Solid Edge part; units mm, degrees
sketch "Sketch1" plane through (0, 0, 0) normal (0, 0, 1) x (1, 0, 0)
  circle A0 centre (0, 0) radius 9.135
extrude "Protrusion1" add sketch "Sketch1" along normal blind 9
sketch "Sketch2" plane through (0, 0, 9) normal (0, 0, 1) x (1, 0, 0)
  line L0 (0, -3.4641) -> (-3, -1.7321)
  line L1 (-3, -1.7321) -> (-3, 1.7321)
  line L2 (-3, 1.7321) -> (0, 3.4641)
  line L3 (0, 3.4641) -> (3, 1.7321)
  line L4 (3, 1.7321) -> (3, -1.7321)
  line L5 (3, -1.7321) -> (0, -3.4641)
extrude "Cutout1" cut sketch "Sketch2" against normal blind 4.5
sketch "Sketch3" plane through (0, 0, 0) normal (0, 0, -1) x (0, 1, 0)
  circle A0 centre (0, 0) radius 6
extrude "Protrusion2" add sketch "Sketch3" along normal blind 25
sketch "Sketch4" plane through (0, 0, -25) normal (0, 0, -1) x (0, 1, 0)
  circle A0 centre (0, 0) radius 5
extrude "Protrusion3" add sketch "Sketch4" along normal blind 16
chamfer "Chamfer1" distance 0.5 angle 45 1 edges at (0, -5, -41)
properties part number "142603"
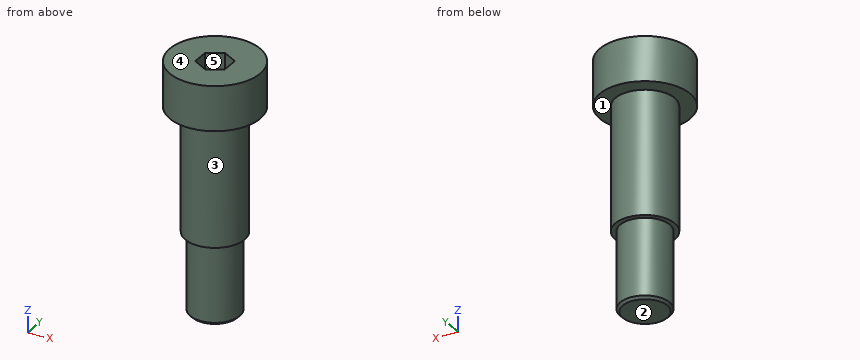
Check sheet for the modelled part. Datum: model origin and axes. Units: mm. Face numbers are marked on the shaded views. A direction names the side the tool comes from. Coordinates: 2 decimals unless noted, no trailing zeros. Write each loop counter-clockwise with the first axis right and the second up, starting at its lowest first coordinate (ties: lowest second). Pieces come first, ordered by that corner, then holes. Notation, with made-up numbers: (67.5, -16) - (76.5, -16) arc R13 cw to (76.5, -1) - close; hole circle Ø2 at (87, 46). An arc over 180 degrees is marked (long way). One line per question, with ' | ' between items.
Item 1: Gauge pin test, flat ends, axial feed: P1, Ø1.5, axis at x = 1, z = -12, coming from the -Y side; P2, Ø3, axis at y = 1.5, z = -9, coming from the -X side; P3, Ø3, axis at y = -0.5, z = 6.5, coming from the -X side (3 decimals); P4, Ø10, axis at x = 5.5, z = -34, coming from the -Y side. Record the tip position at first contact, or that the pin passes through.
Determined:
P1: stops at y = -5.99 | P2: stops at x = -6 | P3: stops at x = -9.135 | P4: stops at y = -4.97
Item 2: Sectioned sample at D-D on y = -7. Record the boundary of the cut face in (x, z), plus the area to 3 significant figures.
Determined:
outline: (-5.87, 0) - (5.87, 0) - (5.87, 9) - (-5.87, 9) - close | area: 106 mm2
Item 3: Sectioned sample at A-A on y = 0. Record the boundary of the cut face in (x, z) (3 decimals), plus the area to 3 significant figures.
Determined:
outline: (-9.135, 0) - (-6, 0) - (-6, -25) - (-5, -25) - (-5, -40.5) - (-4.5, -41) - (4.5, -41) - (5, -40.5) - (5, -25) - (6, -25) - (6, 0) - (9.135, 0) - (9.135, 9) - (3, 9) - (3, 4.5) - (-3, 4.5) - (-3, 9) - (-9.135, 9) - close | area: 597 mm2
Item 4: Thickness scan on line 1 (Z direction, x = 4, y = 5.5); line 2 (Z direction, x = 0.25, y = 3); line 3 (Y direction, x = -0.5, z = -30). Record the ranges inside material, lowest first. Write a range as [from, to].
Determined:
line 1: z = [0, 9] | line 2: z = [-41, 4.5] | line 3: y = [-4.97, 4.97]
Item 5: Sectioned sample at B-B on z = -25.5. Record the boundary of the cut face in (x, y).
Determined:
outline: circle Ø10 at (0, 0)
Item 6: Access from +Z, -Z, +X, -X, +Y, -Y to the whole of each face (thin tool, end or side, straight path). Record for the marked faces 1 and 2.
Determined:
face 1: -Z | face 2: -Z, +X, -X, +Y, -Y
Item 7: Sectioned sample at C-C on z = -17. Record the boundary of the cut face in (x, y), plus the area to 3 significant figures.
Determined:
outline: circle Ø12 at (0, 0) | area: 113 mm2
Item 8: Mould release check, pull along X, two halves, no side actions. Record for the marked faces 3, 4 and 5: pulls with the +X half, pulls with the -X half, needs draft (parallel to the pull), parting line crosses it, or undercut.
Determined:
face 3: parting line crosses it | face 4: needs draft | face 5: undercut
